```python
from build123d import *

# Parameters (mm, degrees)
SKETCH1_W           = 11
SKETCH1_H           = 8
SKETCH1_R           = 2.5
BOSS_EXTRUDE1_DEPTH = 4.3
CUT_EXTRUDE1_DEPTH  = 9
SKETCH3_W           = 6.77
SKETCH3_H           = 8
SKETCH3_R           = 2.5
BOSS_EXTRUDE2_DEPTH = 1.8
FILLET1_R           = 4
FILLET2_R           = 1


with BuildPart() as part:
    # Sketch1 → Boss-Extrude1 (new body)
    with BuildSketch(Plane(origin=(0, 0, 0), x_dir=(1, 0, 0), z_dir=(0, 1, 0))):
        Rectangle(SKETCH1_W, SKETCH1_H)
        Circle(SKETCH1_R, mode=Mode.SUBTRACT)
    extrude(amount=BOSS_EXTRUDE1_DEPTH)

    # Sketch2 → Cut-Extrude1 (cut, through all)
    with BuildSketch(Plane.XY.offset(4)):
        Polygon((-5.5, 2.66), (-2.84, 0), (-5.5, 0), align=None)
        Polygon((5.5, 2.66), (5.5, 0), (2.84, 0), align=None)
    extrude(amount=-CUT_EXTRUDE1_DEPTH, mode=Mode.SUBTRACT)

    # Sketch3 → Boss-Extrude2 (add)
    with BuildSketch(Plane(origin=(0, 4.3, 0), x_dir=(1, 0, 0), z_dir=(0, 1, 0))):
        Rectangle(SKETCH3_W, SKETCH3_H)
        Circle(SKETCH3_R, mode=Mode.SUBTRACT)
    extrude(amount=BOSS_EXTRUDE2_DEPTH)

    # Fillet1
    fillet1_edges = [part.edges().sort_by_distance(p)[0] for p in [
        (3.385, 5.2, -4),
        (-3.385, 5.2, 4),
    ]]
    fillet(fillet1_edges, radius=FILLET1_R)

    # Fillet2
    fillet2_edges = [part.edges().sort_by_distance(p)[0] for p in [
        (5.5, 3.48, 4),
        (-5.5, 3.48, -4),
    ]]
    fillet(fillet2_edges, radius=FILLET2_R)


solid = part.part
```
Build history of the part. All positions in model axes, mm. A direction names the side the tool comes from. Give positions to 0.01 mm unless a question says otherwise; leave off trailing zeros. Loops run counter-clockwise (first coordinate to the right, second up) from the corner with the lowest first, then second, coordinate; pieces in that order, holes last. Notation, with made-up numbers: (71.5, 10) -> (84.5, 10) arc R17 ccw to (84.5, 23) -> close; hole circle Ø8 at (17.25, 31.5). An arc over 180 degrees is marked (long way). One line per question, with ' | ' between items. Start each with the question number.
1) Pin check, flat tips, straight feed: pin 1 (2 mm diameter, centred on y = 1, z = 3, fed in from +X); pin 2 (4 mm diameter, centred on x = 0, z = 0, fed in from +Y); pin 3 (2 mm diameter, centred on y = 5.5, z = -1.5, fed in from -X) (3 decimals); pin 4 (2 mm diameter, centred on y = 1.5, z = 0.5, fed in from +X). Stop position of each tip, or through.
2) 3-axis set-ups, long thin cutter, end or side, ignore diameter. For faces 4 (the flat face through (4.15, 1.31, 0.06)), 5 (the cylindrical face through (-2.24, 5.21, 2.8)), 6 (the cylindrical face through (2.24, 5.21, -2.8)): which of +Z, -Z, +X, -X, +Y, -Y reach the whole face in a straight line?
3) Probe L1, parallel to Z at x = 0, y = 3; L2, parallel to X at y = 4.25, z = 0; L3, parallel to Y at x = -2.75, z = 2.5. List the from-to ranges inside material, lowest first.
4) Cut at A-A (y = 5). Give the cut face in (x, z) (3 decimals).
5) Cut at C-C (x = -2.25). Give the cut face in (y, z).
6) Two-plate mould, pull along X, no slides. Class faces 1 (the flat face through (3.385, 5, 2)), 2 (the flat face through (-3.385, 5, -2)), 3 (the cylindrical face through (-0.54, 3.01, 2.44)): released by +X, released by -X, zero draft, split by the parting line, or undercut.
7) Cut at D-D (y = 1.25). Give the cut face in (x, z), plus the area to 3 significant figures.
8) Cut at B-B (z = 1). Give the cut face in (x, y) (3 decimals).
Return value:
1) pin 1: x = 4.84 | pin 2: through | pin 3: x = -3.385 | pin 4: x = 5.34
2) face 4: +Z, -Z, +X, -Y | face 5: +Z, -X, +Y | face 6: -Z, +X, +Y
3) L1: -4 to -2.5, 2.5 to 4 | L2: -5.5 to -2.5, 2.5 to 5.5 | L3: 0 to 4.3
4) outline: (-3.385, -4) -> (-0.615, -4) arc R4 ccw to (3.385, 0) -> (3.385, 4) -> (0.615, 4) arc R4 ccw to (-3.385, 0) -> close; hole circle Ø5 at (0, 0)
5) outline: (0, -4) -> (6.1, -4) -> (6.1, -1.09) -> (0, -1.09) -> close; (0, 1.09) -> (6.1, 1.09) -> (6.1, 2.79) -> (4.3, 2.79) -> (4.3, 4) -> (0, 4) -> close
6) face 1: released by +X | face 2: released by -X | face 3: undercut
7) outline: (-4.09, -4) -> (4.09, -4) -> (4.09, 4) -> (-4.09, 4) -> close; hole circle Ø5 at (0, 0) | area: 45.8 mm^2
8) outline: (-5.5, 2.66) -> (-2.84, 0) -> (-2.291, 0) -> (-2.291, 6.1) -> (-3.258, 6.1) -> (-3.258, 4.3) -> (-5.5, 4.3) -> close; (2.291, 0) -> (2.84, 0) -> (5.5, 2.66) -> (5.5, 4.3) -> (3.385, 4.3) -> (3.385, 6.1) -> (2.291, 6.1) -> close
